from build123d import *

# Parameters (mm, degrees)
BODY_DEPTH                             = 70
FRONTAL_M3_NUT_CUTOUTS_DEPTH           = 3
FRONTAL_M4_NUT_CUTOUT_DEPTH            = 4
MAIN_CHAMFER_SIZE                      = 5
SIDE_CHAMFER_SIZE                      = 1
WALL_CHAMFERS_SIZE                     = 10
CLEARANCE_CUTOUT_DEPTH                 = 4
M3_FULL_MIRROR_COPY_3_DEPTH            = 3
BOTTOM_BOARD_MOUNTING_HOLE_D           = 4.5
BOTTOM_BOARD_MOUNTING_HOLE_CBORE_D     = 8
BOTTOM_BOARD_MOUNTING_HOLE_CBORE_DEPTH = 4.4
BOTTOM_M4_NUT_CUTOUT_DEPTH             = 4


# Read off the part's stored shape, not the designer's step: hull_mounting_holes
with BuildPart() as part:
    # body_sketch → body (new body)
    with BuildSketch(Plane(origin=(0, 0, 0), x_dir=(0, 0, -1), z_dir=(1, 0, 0))):
        Polygon((0, 0), (0, 20), (-8, 20), (-8, 55), (-20, 55), (-20, 20), (-55, 20), (-55, 8), (-20, 8), (-20, 0), align=None)
    extrude(amount=BODY_DEPTH)

    # rod_hole_sketch_auto → rod_hole_d10 (revolve, cut)
    with BuildSketch(Plane(origin=(70, 10, 10), x_dir=(0, 0, -1), z_dir=(0, 1, 0))):
        Polygon((0, 0), (0, 70), (5.25, 70), (5.1, 69.740192379), (5.1, 0.259807621), (5.25, 0), align=None)
    revolve(axis=Axis((76.35, 10, 10), (-1, 0, 0)), mode=Mode.SUBTRACT)

    # hull_mounting_holes outline → hull_mounting_holes (revolve, cut)
    with BuildSketch(Plane(origin=(25, 45, 0), x_dir=(1, 0, 0), z_dir=(0, -1, 0))):
        Polygon((0, 8), (1.8, 8), (1.7, 8.1), (1.7, 19.9), (1.8, 20), (0, 20), align=None)
    hull_mounting_holes = revolve(axis=Axis((25, 45, 0), (0, 0, 1)), mode=Mode.SUBTRACT)

    # hull_mounting_holes 2 outline → hull_mounting_holes 2 (revolve, cut)
    with BuildSketch(Plane(origin=(10, 30, 0), x_dir=(1, 0, 0), z_dir=(0, -1, 0))):
        Polygon((0, 8), (1.8, 8), (1.7, 8.1), (1.7, 19.9), (1.8, 20), (0, 20), align=None)
    hull_mounting_holes_2 = revolve(axis=Axis((10, 30, 0), (0, 0, 1)), mode=Mode.SUBTRACT)

    # Sketch8 → board_mounting_hole (revolve, cut)
    with BuildSketch(Plane(origin=(25, 30, 8), x_dir=(0, 1, 0), z_dir=(1, 0, 0))):
        Polygon((0, 0), (0, 12), (2.275, 12), (2.25, 11.975), (2.25, 4.4), (4, 4.4), (4, 0.025), (4.025, 0), align=None)
    board_mounting_hole = revolve(axis=Axis((25, 30, 1.65), (0, 0, 1)), mode=Mode.SUBTRACT)

    # Sketch9 → frontal_m3_nut_cutouts (cut)
    with BuildSketch(Plane.XY.offset(20)):
        Polygon((25, 48.175426481), (22.25, 46.58771324), (22.25, 43.41228676), (25, 41.824573519), (27.75, 43.41228676), (27.75, 46.58771324), align=None)
        Polygon((10, 33.175426481), (7.25, 31.58771324), (7.25, 28.41228676), (10, 26.824573519), (12.75, 28.41228676), (12.75, 31.58771324), align=None)
    frontal_m3_nut_cutouts = extrude(amount=-FRONTAL_M3_NUT_CUTOUTS_DEPTH, mode=Mode.SUBTRACT)

    # Sketch10 → frontal_m4_nut_cutout (cut)
    with BuildSketch(Plane.XY.offset(20)):
        Polygon((21.5, 32.020725942), (21.5, 27.979274058), (25, 25.958548116), (28.5, 27.979274058), (28.5, 32.020725942), (25, 34.041451884), align=None)
    frontal_m4_nut_cutout = extrude(amount=-FRONTAL_M4_NUT_CUTOUT_DEPTH, mode=Mode.SUBTRACT)

    # frontal_m4_mirror: board_mounting_hole, frontal_m4_nut_cutout across plane
    add(board_mounting_hole.mirror(Plane.ZY.offset(-35)), mode=Mode.SUBTRACT)
    add(frontal_m4_nut_cutout.mirror(Plane.ZY.offset(-35)), mode=Mode.SUBTRACT)

    # main_chamfer
    main_chamfer_edges = [part.edges().sort_by_distance(p)[0] for p in [
        (35, 0, 0),
    ]]
    chamfer(main_chamfer_edges, length=MAIN_CHAMFER_SIZE)

    # side_chamfer
    side_chamfer_edges = [part.edges().sort_by_distance(p)[0] for p in [
        (0, 4, 20),
        (70, 20, 4),
        (0, 20, 4),
        (0, 0, 12.5),
        (0, 12.5, 0),
        (70, 12.5, 0),
        (0, 2.5, 2.5),
        (70, 2.5, 2.5),
        (35, 0, 20),
        (35, 20, 0),
        (70, 4, 20),
        (70, 0, 12.5),
    ]]
    chamfer(side_chamfer_edges, length=SIDE_CHAMFER_SIZE)

    # wall_chamfers
    wall_chamfers_edges = [part.edges().sort_by_distance(p)[0] for p in [
        (0, 14, 55),
        (0, 55, 14),
        (70, 55, 14),
        (70, 14, 55),
    ]]
    chamfer(wall_chamfers_edges, length=WALL_CHAMFERS_SIZE)

    # Sketch11 → clearance_cutout (cut)
    with BuildSketch(Plane.XY.offset(20)):
        Polygon((0, 20), (5, 20), (5, 40), (15, 50), (55, 50), (65, 40), (65, 20), (70, 20), (70, 45), (60, 55), (10, 55), (0, 45), align=None)
    extrude(amount=-CLEARANCE_CUTOUT_DEPTH, mode=Mode.SUBTRACT)

    # bottom_m3_mirror: hull_mounting_holes, hull_mounting_holes 2, frontal_m3_nut_cutouts across plane
    add(hull_mounting_holes.mirror(Plane(origin=(0, 0, 0), x_dir=(0, 0.7071067811865476, 0.7071067811865475), z_dir=(0, 0.7071067811865475, -0.7071067811865476))), mode=Mode.SUBTRACT)
    add(hull_mounting_holes_2.mirror(Plane(origin=(0, 0, 0), x_dir=(0, 0.7071067811865476, 0.7071067811865475), z_dir=(0, 0.7071067811865475, -0.7071067811865476))), mode=Mode.SUBTRACT)
    add(frontal_m3_nut_cutouts.mirror(Plane(origin=(0, 0, 0), x_dir=(0, 0.7071067811865476, 0.7071067811865475), z_dir=(0, 0.7071067811865475, -0.7071067811865476))), mode=Mode.SUBTRACT)

    # m3_full_mirror: hull_mounting_holes, hull_mounting_holes 2, frontal_m3_nut_cutouts across plane
    add(hull_mounting_holes.mirror(Plane.ZY.offset(-35)), mode=Mode.SUBTRACT)
    add(hull_mounting_holes_2.mirror(Plane.ZY.offset(-35)), mode=Mode.SUBTRACT)
    add(frontal_m3_nut_cutouts.mirror(Plane.ZY.offset(-35)), mode=Mode.SUBTRACT)

    # m3_full_mirror copy 1 sketch → m3_full_mirror copy 1 (revolve, cut)
    with BuildSketch(Plane(origin=(45, 0, 45), x_dir=(-1, 0, 0), z_dir=(0, 0, -1))):
        Polygon((0, 8), (1.8, 8), (1.7, 8.1), (1.7, 19.9), (1.8, 20), (0, 20), align=None)
    revolve(axis=Axis((45, 0, 45), (0, 1, 0)), mode=Mode.SUBTRACT)

    # m3_full_mirror copy 2 sketch → m3_full_mirror copy 2 (revolve, cut)
    with BuildSketch(Plane(origin=(60, 0, 30), x_dir=(-1, 0, 0), z_dir=(0, 0, -1))):
        Polygon((0, 8), (1.8, 8), (1.7, 8.1), (1.7, 19.9), (1.8, 20), (0, 20), align=None)
    revolve(axis=Axis((60, 0, 30), (0, 1, 0)), mode=Mode.SUBTRACT)

    # m3_full_mirror copy 3 sketch → m3_full_mirror copy 3 (cut)
    with BuildSketch(Plane(origin=(70, 20, 0), x_dir=(-1, 0, 0), z_dir=(0, 1, 0))):
        Polygon((25, 48.175426481), (22.25, 46.58771324), (22.25, 43.41228676), (25, 41.824573519), (27.75, 43.41228676), (27.75, 46.58771324), align=None)
        Polygon((10, 33.175426481), (7.25, 31.58771324), (7.25, 28.41228676), (10, 26.824573519), (12.75, 28.41228676), (12.75, 31.58771324), align=None)
    extrude(amount=-M3_FULL_MIRROR_COPY_3_DEPTH, mode=Mode.SUBTRACT)

    # m3_full_mirror copy 4 sketch → m3_full_mirror copy 4 (revolve, cut)
    with BuildSketch(Plane(origin=(60, 30, 0), x_dir=(-1, 0, 0), z_dir=(0, -1, 0))):
        Polygon((0, -8), (1.8, -8), (1.7, -8.1), (1.7, -19.9), (1.8, -20), (0, -20), align=None)
    revolve(axis=Axis((60, 30, 0), (0, 0, -1)), mode=Mode.SUBTRACT)

    # bottom_board_mounting_hole (through all)
    with Locations(Plane.XZ.offset(-8)):
        with Locations((10, 45)):
            bottom_board_mounting_hole = CounterBoreHole(BOTTOM_BOARD_MOUNTING_HOLE_D / 2, BOTTOM_BOARD_MOUNTING_HOLE_CBORE_D / 2, BOTTOM_BOARD_MOUNTING_HOLE_CBORE_DEPTH)

    # Sketch15 → bottom_m4_nut_cutout (cut)
    with BuildSketch(Plane(origin=(0, 20, 0), x_dir=(1, 0, 0), z_dir=(0, 1, 0))):
        Polygon((10, -40.958548116), (6.5, -42.979274058), (6.5, -47.020725942), (10, -49.041451884), (13.5, -47.020725942), (13.5, -42.979274058), align=None)
    bottom_m4_nut_cutout = extrude(amount=-BOTTOM_M4_NUT_CUTOUT_DEPTH, mode=Mode.SUBTRACT)

    # bottom_m4_mirror: bottom_board_mounting_hole, bottom_m4_nut_cutout across plane
    add(bottom_board_mounting_hole.mirror(Plane.ZY.offset(-35)), mode=Mode.SUBTRACT)
    add(bottom_m4_nut_cutout.mirror(Plane.ZY.offset(-35)), mode=Mode.SUBTRACT)


solid = part.part
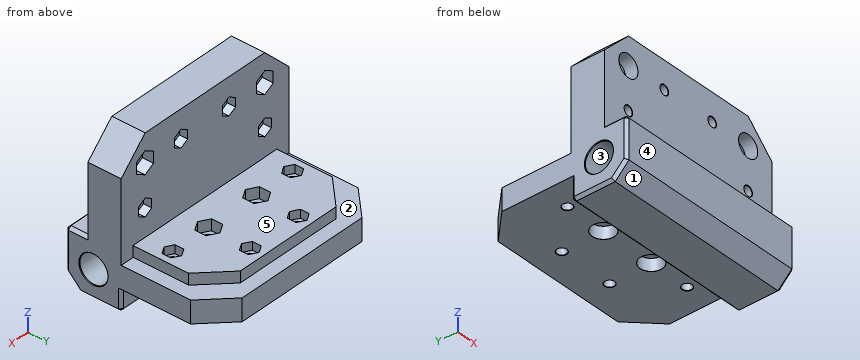
Work out the finished part from the listing and answer in its coordinate system (mm). Face numbers are marked on the shaded views. A direction names the side the tool comes from. Round coordinates to 2 decimals unless told otherwise and drop trailing zeros. Write each loop counter-clockwise with the first axis right and the second up, starting at its lowest first coordinate (ties: lowest second). Pieces come first, ordered by that corner, then holes. Notation, with made-up numbers: M 45.5,-24.75 L 103.5,-24.75 A26 cw 103.5,-0.75 Z; hole C 32.25,8.5 d5. An arc over 180 degrees is marked long. Use a Markdown table: item, result.
1) Determine the mould class of the marked faces 3, 4 and 5 for opening direction Y: pulls with the +Y half, pulls with the -Y half, needs draft (parallel to the pull), parting line crosses it, or undercut.
Taken from the geometry:
| item | result |
|---|---|
| face 3 | undercut |
| face 4 | pulls with the -Y half |
| face 5 | needs draft |
2) Which of the six approach directions +Z, -Z, +X, -X, +Y, -Y give full straight-line access (tool end or side, diameter ignored) to the marked faces 1 and 2?
Taken from the geometry:
| item | result |
|---|---|
| face 1 | -Z, +X, -X, -Y |
| face 2 | +Z, +Y |
3) The part is cut by section D-D on z = 30. Give the vertices of the cut face in (x, y), plus the area to 3 significant figures.
Taken from the geometry:
| item | result |
|---|---|
| outline | M 0,8 L 8.2,8 L 8.3,8.1 L 8.3,17 L 7.25,17 L 7.25,20 L 0,20 Z; M 11.7,8.1 L 11.8,8 L 58.2,8 L 58.3,8.1 L 58.3,17 L 57.25,17 L 57.25,20 L 12.75,20 L 12.75,17 L 11.7,17 Z; M 61.7,8.1 L 61.8,8 L 70,8 L 70,20 L 62.75,20 L 62.75,17 L 61.7,17 Z |
| area | 746 mm2 |
4) Consider line 1 (Z direction, x = 10, y = 10); line 2 (Z direction, x = 28.5, y = 11); line 3 (Y direction, x = 11, z = 42). Determine where each line is inside the solid, lowest interval first. Write a range as [from, to].
Taken from the geometry:
| item | result |
|---|---|
| line 1 | z = [0, 4.9], [15.1, 28.3], [31.7, 41], [49, 55] |
| line 2 | z = [0, 5], [15, 55] |
| line 3 | y = [12.4, 16] |
5) The part is cut by section B-B on y = 10. Give the vertices of the cut face in (x, z).
Taken from the geometry:
| item | result |
|---|---|
| outline | M 0,1 L 1,0 L 69,0 L 70,1 L 70,4.75 L 69.74,4.9 L 0.26,4.9 L 0,4.75 Z; M 0,15.25 L 0.26,15.1 L 69.74,15.1 L 70,15.25 L 70,45 L 60,55 L 10,55 L 0,45 Z; hole C 10,45 d8; hole C 10,30 d3.4; hole C 25,45 d3.4; hole C 45,45 d3.4; hole C 60,45 d8; hole C 60,30 d3.4 |
6) The part is cut by section C-C on x = 32. Give the vertices of the cut face in (y, z), plus the area to 3 significant figures.
Taken from the geometry:
| item | result |
|---|---|
| outline | M 0,5 L 5,0 L 19,0 L 20,1 L 20,8 L 55,8 L 55,16 L 50,16 L 50,20 L 20,20 L 20,55 L 8,55 L 8,20 L 1,20 L 0,19 Z; hole C 10,10 d10.2 |
| area | 1,120 mm2 |
7) Flat-ended cylindrical pins translate along their axes: pin 1 (6 mm diameter, centred on x = 25, y = 30, fed in from +Z); pin 2 (12 mm diameter, centred on x = 52, y = 40, fed in from +Z); pin 3 (6 mm diameter, centred on x = 10, z = 30.5, fed in from +Y). Find the tip coordinate at first contact, or state that the pin passes through.
Taken from the geometry:
| item | result |
|---|---|
| pin 1 | stops at z = 16 |
| pin 2 | stops at z = 20 |
| pin 3 | stops at y = 20 |
8) The part is cut by section A-A on z = 10. Give the vertices of the cut face in (x, y).
Taken from the geometry:
| item | result |
|---|---|
| outline | M 0,1 L 1,0 L 69,0 L 70,1 L 70,4.75 L 69.74,4.9 L 0.26,4.9 L 0,4.75 Z; M 0,15.25 L 0.26,15.1 L 69.74,15.1 L 70,15.25 L 70,45 L 60,55 L 10,55 L 0,45 Z; hole C 10,30 d3.4; hole C 25,30 d8; hole C 25,45 d3.4; hole C 45,30 d8; hole C 45,45 d3.4; hole C 60,30 d3.4 |
